```python
from build123d import *

# Parameters (mm, degrees)
SKETCH_1_R          = 55
EXTRUDE_1_DEPTH     = 150
SKETCH_2_R          = 50
CUT_EXTRUDE_1_DEPTH = 145
SKETCH_3_R          = 13.75
CUT_EXTRUDE_2_DEPTH = 169.967452487


with BuildPart() as part:
    # 草图1 → 拉伸1 (new body)
    with BuildSketch(Plane(origin=(0, 0, 0), x_dir=(1, 0, 0), z_dir=(0, 1, 0))):
        with Locations(Location((0, 0, 0), (0, 0, 270))):
            Circle(SKETCH_1_R)
    extrude(amount=EXTRUDE_1_DEPTH)

    # 草图2 → 切除-拉伸1 (cut)
    with BuildSketch(Plane(origin=(0, 150, 0), x_dir=(-1, 0, 0), z_dir=(0, 1, 0))):
        with Locations(Location((0, 0, 0), (0, 0, 90))):
            Circle(SKETCH_2_R)
    extrude(amount=-CUT_EXTRUDE_1_DEPTH, mode=Mode.SUBTRACT)

    # 草图3 → 切除-拉伸2 (cut, through all)
    with BuildSketch(Plane.XZ):
        with Locations(Location((0, 0, 0), (0, 0, 270))):
            Circle(SKETCH_3_R)
    extrude(amount=-CUT_EXTRUDE_2_DEPTH, mode=Mode.SUBTRACT)


solid = part.part
```
Here's how the part is built. I have some questions about the finished solid (model axes, mm). A direction names the side the tool comes from. Round coordinates to 2 decimals unless told otherwise and drop trailing zeros. Loops run counter-clockwise (first coordinate to the right, second up) from the corner with the lowest first, then second, coordinate; pieces in that order, holes last. Notation, with made-up numbers: (17, -36) -> (75, -36) arc R25 cw to (75, -15) -> close; hole circle Ø11 at (40, -21). An arc over 180 degrees is marked (long way). Answer as CSV lines item,"result". Start each with the question number.
1. For faces 1 (the face through (15.02, 78.52, 47.69)), 2 (the face through (-49, 150, 12)), which set-ups out of +Z, -Z, +X, -X, +Y, -Y let a thin tool reach every point of the face, with its end or its side?
2. I'm going to push flat-ended pins straight in: P1, Ø8, axis at x = -6, z = 10.5, coming from the +Y side; P2, Ø5, axis at x = -40, y = 18, coming from the +Z side; P3, Ø5, axis at y = 84, z = 41.5, coming from the +X side. Where does each tip first touch, or does it pass through?
3. If we mould it in two halves opening along X, with no side actions, what happens to faces 3 (the face through (-10, 5, 10)), 4 (the face through (-11, 0, 11)), 5 (the face through (-48.794, 73.95, 25.379))? For each: pulls with the +X half, pulls with the -X half, needs draft (parallel to the pull), parting line crosses it, or undercut.
4. Imagine slicing it at C-C on x = -30.5. Write out the boundary of the cut face in (y, z).
5. I need wall thicknesses on probe 1 along X at (y, z) = (2, 0); probe 2 along Y at (x, z) = (-1, -38.5); probe 3 along Z at (x, y) = (35, 18). Which ranges of each line are inside material? Lowest first, please. Write a range as from..to.
6. Imagine slicing it at D-D on y = 95. Write out the boundary of the cut face in (x, z).
7. Imagine slicing it at A-A on x = 0. Write out the boundary of the cut face in (y, z), plus the area to 3 significant figures.
8. Imagine slicing it at B-B on z = 0. Write out the boundary of the cut face in (x, y), plus the area to 3 significant figures.
Solution:
1,face 1,"+Y"
1,face 2,"+Z, -Z, +X, -X, +Y"
2,P1,"y = 5"
2,P2,"z = 40.23"
2,P3,"x = 38.78"
3,face 3,"undercut"
3,face 4,"needs draft"
3,face 5,"parting line crosses it"
4,outline,"(0, -45.77) -> (150, -45.77) -> (150, -39.62) -> (5, -39.62) -> (5, 39.62) -> (150, 39.62) -> (150, 45.77) -> (0, 45.77) -> close"
5,probe 1,"-55..-13.75, 13.75..55"
5,probe 2,"0..5"
5,probe 3,"-42.43..-35.71, 35.71..42.43"
6,outline,"circle Ø110 at (0, 0); hole circle Ø100 at (0, 0)"
7,outline,"(0, -55) -> (150, -55) -> (150, -50) -> (5, -50) -> (5, -13.75) -> (0, -13.75) -> close; (0, 13.75) -> (5, 13.75) -> (5, 50) -> (150, 50) -> (150, 55) -> (0, 55) -> close"
7,area,"1,860 mm²"
8,outline,"(-55, 0) -> (-13.75, 0) -> (-13.75, 5) -> (-50, 5) -> (-50, 150) -> (-55, 150) -> close; (13.75, 0) -> (55, 0) -> (55, 150) -> (50, 150) -> (50, 5) -> (13.75, 5) -> close"
8,area,"1,860 mm²"
